Here's how the part is built. I have some questions about the finished solid (model axes, mm). Give positions to 0.01 mm unless a question says otherwise; leave off trailing zeros. Write each loop counter-clockwise with the first axis right and the second up, starting at its lowest first coordinate (ties: lowest second). Pieces come first, ordered by that corner, then holes. Notation, with made-up numbers: M -31.5,18 L 22.5,18 A11 ccw 22.5,33 Z; hole C 29.25,-16.75 d6. An arc over 180 degrees is marked long. Answer as CSV lines item,"result". Start each with the question number.
Q1. Suppose I cut it at C-C (y = 1.9). Count the separate pieces of the cut face and the enclosed holes in it, then the cut area to 3 significant figures.
Q2. If I drill on line 1 along X through (y, z) = (0.8, 0.5); line 2 along X through (y, z) = (4.5, 41), over which ranges is the centre line in solid material (lowest first)?
Q3. Suppose I cut it at B-B (x = -22.5). Write out the boundary of the cut face in (y, z), then the cut area to 3 significant figures.
Q4. Suppose I cut it at D-D (x = 37). Write out the boundary of the cut face in (y, z), then the cut area to 3 significant figures.
Q5. Suppose I cut it at A-A (z = 0). Write out the boundary of the cut face in (x, y).
Q6. For pin 1 (1.5 mm diameter, centred on y = 1.5, z = -50, fed in from +X); pin 2 (1 mm diameter, centred on y = 2, z = 3.5, fed in from -X); pin 3 (3 mm diameter, centred on y = 2, z = -5.5, fed in from +X), each with a flat end and sliding along its axis, tell me the tip position at first contact or that it passes through.
Autodesk Inventor part; units mm, degrees
ref_plane "YZ Plane" through (0, 0, 0) normal (1, 0, 0) x (0, 1, 0)
ref_plane "XZ Plane" through (0, 0, 0) normal (0, 1, 0) x (-1, 0, 0)
ref_plane "XY Plane" through (0, 0, 0) normal (0, 0, 1) x (1, 0, 0)
sketch "Sketch1" plane through (0, 0, 0) normal (0, 1, 0) x (-1, 0, 0)
  circle A0 centre (0, 0) radius 75
  circle A1 centre (0, 0) radius 33
  circle A2 centre (55, 0) radius 4.25
  circle A3 centre (38.8909, 38.8909) radius 4.25
  circle A4 centre (0, 55) radius 4.25
  circle A5 centre (-38.8909, 38.8909) radius 4.25
  circle A6 centre (-55, 0) radius 4.25
  circle A7 centre (-38.8909, -38.8909) radius 4.25
  circle A8 centre (0, -55) radius 4.25
  circle A9 centre (38.8909, -38.8909) radius 4.25
  dimension "d0" = 150
  dimension "d1" = 66
  dimension "d2" = 55
  dimension "d3" = 8.5
  dimension "d6" = 360
extrude "Extrusion1" add sketch "Sketch1" along normal blind 5
properties part number "plateHole" material "Steel"
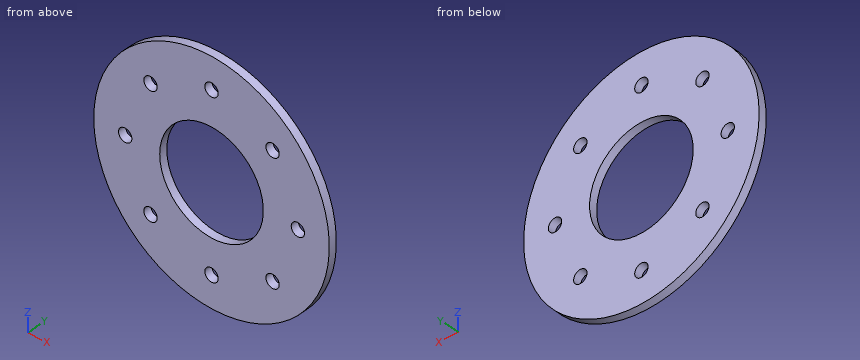
Resolved:
1,separate pieces,"1"
1,enclosed holes,"9"
1,area,"13,800 mm^2"
2,line 1,"-75 to -59.22, -50.78 to -33, 33 to 50.78, 59.22 to 75"
2,line 2,"-62.8 to -42.58, -35.2 to 35.2, 42.58 to 62.8"
3,outline,"M 0,-71.55 L 5,-71.55 L 5,-24.14 L 0,-24.14 Z; M 0,24.14 L 5,24.14 L 5,71.55 L 0,71.55 Z"
3,area,"474 mm^2"
4,outline,"M 0,-65.24 L 5,-65.24 L 5,-42.7 L 0,-42.7 Z; M 0,-35.08 L 5,-35.08 L 5,35.08 L 0,35.08 Z; M 0,42.7 L 5,42.7 L 5,65.24 L 0,65.24 Z"
4,area,"576 mm^2"
5,outline,"M -75,0 L -59.25,0 L -59.25,5 L -75,5 Z; M -50.75,0 L -33,0 L -33,5 L -50.75,5 Z; M 33,0 L 50.75,0 L 50.75,5 L 33,5 Z; M 59.25,0 L 75,0 L 75,5 L 59.25,5 Z"
6,pin 1,"x = 56.56"
6,pin 2,"x = -74.94"
6,pin 3,"x = 74.89"
